Source: CAD feature listing. Evaluate the final solid. Frame: model axes, mm. Give positions to 0.01 mm unless a question says otherwise; leave off trailing zeros. Write each loop counter-clockwise with the first axis right and the second up, starting at its lowest first coordinate (ties: lowest second). Pieces come first, ordered by that corner, then holes. Notation, with made-up numbers: M -6.5,-8 L 22.5,-8 A24 ccw 22.5,24 Z; hole C 13,5.25 d3. An arc over 180 degrees is marked long. Return JSON: item names as keys, results as strings.
```python
from build123d import *

# Parameters (mm, degrees)
SKETCH1_W           = 50.8
SKETCH1_H           = 50.8
SKETCH1_R           = 1.397
BOSS_EXTRUDE1_DEPTH = 2.54
FILLET1_R           = 5.08


with BuildPart() as part:
    # Sketch1 → Boss-Extrude1 (new body)
    with BuildSketch(Plane.XY):
        with Locations((19.05, -19.05)):
            Rectangle(SKETCH1_W, SKETCH1_H)
        Circle(SKETCH1_R, mode=Mode.SUBTRACT)
        with Locations((12.7, 0)):
            Circle(SKETCH1_R, mode=Mode.SUBTRACT)
        with Locations((25.4, 0)):
            Circle(SKETCH1_R, mode=Mode.SUBTRACT)
        with Locations((38.1, 0)):
            Circle(SKETCH1_R, mode=Mode.SUBTRACT)
        with Locations((12.7, -12.7)):
            Circle(SKETCH1_R, mode=Mode.SUBTRACT)
        with Locations((25.4, -12.7)):
            Circle(SKETCH1_R, mode=Mode.SUBTRACT)
        with Locations((38.1, -12.7)):
            Circle(SKETCH1_R, mode=Mode.SUBTRACT)
        with Locations((12.7, -25.4)):
            Circle(SKETCH1_R, mode=Mode.SUBTRACT)
        with Locations((25.4, -25.4)):
            Circle(SKETCH1_R, mode=Mode.SUBTRACT)
        with Locations((38.1, -25.4)):
            Circle(SKETCH1_R, mode=Mode.SUBTRACT)
        with Locations((12.7, -38.1)):
            Circle(SKETCH1_R, mode=Mode.SUBTRACT)
        with Locations((25.4, -38.1)):
            Circle(SKETCH1_R, mode=Mode.SUBTRACT)
        with Locations((38.1, -38.1)):
            Circle(SKETCH1_R, mode=Mode.SUBTRACT)
        with Locations((0, -12.7)):
            Circle(SKETCH1_R, mode=Mode.SUBTRACT)
        with Locations((0, -25.4)):
            Circle(SKETCH1_R, mode=Mode.SUBTRACT)
        with Locations((0, -38.1)):
            Circle(SKETCH1_R, mode=Mode.SUBTRACT)
    extrude(amount=BOSS_EXTRUDE1_DEPTH)

    # Fillet1
    fillet1_edges = [part.edges().sort_by_distance(p)[0] for p in [
        (-6.35, 6.35, 1.27),
        (44.45, 6.35, 1.27),
        (44.45, -44.45, 1.27),
        (-6.35, -44.45, 1.27),
    ]]
    fillet(fillet1_edges, radius=FILLET1_R)


solid = part.part
```
1) Cut plane B-B, the plane y = -12.7. Return the cut outline in (x, z), then the cut area to 3 significant figures.
Numbers:
{"outline": "M -6.35,0 L -1.4,0 L -1.4,2.54 L -6.35,2.54 Z; M 1.4,0 L 11.3,0 L 11.3,2.54 L 1.4,2.54 Z; M 14.1,0 L 24,0 L 24,2.54 L 14.1,2.54 Z; M 26.8,0 L 36.7,0 L 36.7,2.54 L 26.8,2.54 Z; M 39.5,0 L 44.45,0 L 44.45,2.54 L 39.5,2.54 Z", "area": "101 mm²"}
2) Contact query for a flat-ended pin moving along its axis: pin 1 Ø2 at (x, y) = (0, -12.7) entering from -Z. Output: stop coordinate, or through.
Numbers:
{"pin 1": "passes through"}
3) Draft query along Y for faces 1 (the face through (24.29, -26.25, 1.25)), 2 (the face through (42.922, 4.901, 1.288)), 3 (the face through (19, -19, 2.54)). Return one class per face: released by +Y, released by -Y, zero draft, split by the parting line, or undercut.
Numbers:
{"face 1": "undercut", "face 2": "released by +Y", "face 3": "zero draft"}
4) Line query: line 1 (Y direction, x = 25.4, z = 0.8); line 2 (X direction, y = -0.5, z = 1); line 3 (Y direction, x = 37.5, z = 2.2). Output: solid intervals per line, ascending. Write a range as [from, to].
Numbers:
{"line 1": "y = [-44.45, -39.5], [-36.7, -26.8], [-24, -14.1], [-11.3, -1.4], [1.4, 6.35]", "line 2": "x = [-6.35, -1.3], [1.3, 11.4], [14, 24.1], [26.7, 36.8], [39.4, 44.45]", "line 3": "y = [-44.45, -39.36], [-36.84, -26.66], [-24.14, -13.96], [-11.44, -1.26], [1.26, 6.35]"}
5) Cut plane A-A, the plane x = 38.1. Return the cut outline in (y, z).
Numbers:
{"outline": "M -44.45,0 L -39.5,0 L -39.5,2.54 L -44.45,2.54 Z; M -36.7,0 L -26.8,0 L -26.8,2.54 L -36.7,2.54 Z; M -24,0 L -14.1,0 L -14.1,2.54 L -24,2.54 Z; M -11.3,0 L -1.4,0 L -1.4,2.54 L -11.3,2.54 Z; M 1.4,0 L 6.35,0 L 6.35,2.54 L 1.4,2.54 Z"}
6) Cut plane C-C, the plane z = 0.9. Give the number of separate pieces and of enclosed holes in the cut face, then the cut area to 3 significant figures.
Numbers:
{"separate pieces": "1", "enclosed holes": "16", "area": "2,460 mm²"}
